```python
from build123d import *

# Parameters (mm, degrees)
F1_DEPTH = 9.525
F2_R     = 3.90906
F3_DEPTH = 25.4
F4_DEPTH = 25.4
F5_R     = 3.90525
F6_DEPTH = 25.4


# Not quite as in the source:
# - a fillet or chamfer that OpenCascade refuses, or shapes differently, is made with other operations: its cross-section is extruded or revolved along the edge and cut away or added


with BuildPart() as f1:
    # F0 (on Top) → F1 (new body, symmetric)
    with BuildSketch(Plane.XY):
        with BuildLine():
            Line((0, 20.6466445854), (-11.58875, 20.6466445854))
            ThreePointArc((-11.58875, 20.6466445854), (-17.1096965819, 19.861848606), (-22.19325, 17.5696355848))
            Line((-22.19325, 17.5696355848), (-22.19325, -17.5696355848))
            ThreePointArc((-22.19325, -17.5696355848), (-17.1096965819, -19.861848606), (-11.58875, -20.6466445854))
            Line((-11.58875, -20.6466445854), (0, -20.6466445854))
            Line((0, -20.6466445854), (11.58875, -20.6466445854))
            ThreePointArc((11.58875, -20.6466445854), (17.1096965819, -19.861848606), (22.19325, -17.5696355848))
            Line((22.19325, -17.5696355848), (22.19325, 17.5696355848))
            ThreePointArc((22.19325, 17.5696355848), (17.1096965819, 19.861848606), (11.58875, 20.6466445854))
            Line((11.58875, 20.6466445854), (0, 20.6466445854))
        make_face()
        with BuildLine():
            ThreePointArc((11.58875, 19.8846445854), (16.6970877606, 19.1869573913), (21.43125, 17.145))
            Line((21.43125, 17.145), (21.43125, -17.145))
            ThreePointArc((21.43125, -17.145), (16.6970877606, -19.1869573913), (11.58875, -19.8846445854))
            Line((11.58875, -19.8846445854), (0, -19.8846445854))
            Line((0, -19.8846445854), (-11.58875, -19.8846445854))
            ThreePointArc((-11.58875, -19.8846445854), (-16.6970877606, -19.1869573913), (-21.43125, -17.145))
            Line((-21.43125, -17.145), (-21.43125, 17.145))
            ThreePointArc((-21.43125, 17.145), (-16.6970877606, 19.1869573913), (-11.58875, 19.8846445854))
            Line((-11.58875, 19.8846445854), (0, 19.8846445854))
            Line((0, 19.8846445854), (11.58875, 19.8846445854))
        make_face(mode=Mode.SUBTRACT)
    extrude(amount=F1_DEPTH, both=True)

    # F2 (on face) → F3 (cut)
    with BuildSketch(Plane.YZ.offset(22.19325)):
        with BuildLine():
            ThreePointArc((0.396875, -6.3375855209), (4.6283180665, -4.3475478002), (6.35, 0))
            ThreePointArc((6.35, 0), (4.6283180665, 4.3475478002), (0.396875, 6.3375855209))
            Line((0.396875, 6.3375855209), (0.396875, -6.3375855209))
        make_face()
        with BuildLine():
            Line((0.396875, -6.3375855209), (0.396875, 6.3375855209))
            ThreePointArc((0.396875, 6.3375855209), (0, 6.35), (-0.396875, 6.3375855209))
            Line((-0.396875, 6.3375855209), (-0.396875, -6.3375855209))
            ThreePointArc((-0.396875, -6.3375855209), (0, -6.35), (0.396875, -6.3375855209))
        make_face()
        with BuildLine():
            ThreePointArc((-0.396875, 6.3375855209), (0, 6.35), (0.396875, 6.3375855209))
            Line((0.396875, 6.3375855209), (0.396875, 16.235569492))
            Line((0.396875, 16.235569492), (-0.396875, 16.235569492))
            Line((-0.396875, 16.235569492), (-0.396875, 6.3375855209))
        make_face()
        with BuildLine():
            Line((0.396875, -16.235569492), (0.396875, -6.3375855209))
            ThreePointArc((0.396875, -6.3375855209), (0, -6.35), (-0.396875, -6.3375855209))
            Line((-0.396875, -6.3375855209), (-0.396875, -16.235569492))
            Line((-0.396875, -16.235569492), (0.396875, -16.235569492))
        make_face()
        with BuildLine():
            Line((-0.396875, -6.3375855209), (-0.396875, 6.3375855209))
            ThreePointArc((-0.396875, 6.3375855209), (-6.35, 0), (-0.396875, -6.3375855209))
        make_face()
        with Locations((-11.9634, 0)):
            Circle(F2_R)
        with Locations((11.9634, 0)):
            Circle(F2_R)
    extrude(amount=-F3_DEPTH, mode=Mode.SUBTRACT)

    # F2 (on face) → F4 (cut)
    with BuildSketch(Plane.YZ.offset(22.19325)):
        with BuildLine():
            ThreePointArc((0.396875, -6.3375855209), (4.6283180665, -4.3475478002), (6.35, 0))
            ThreePointArc((6.35, 0), (4.6283180665, 4.3475478002), (0.396875, 6.3375855209))
            Line((0.396875, 6.3375855209), (0.396875, -6.3375855209))
        make_face()
        with BuildLine():
            Line((0.396875, -6.3375855209), (0.396875, 6.3375855209))
            ThreePointArc((0.396875, 6.3375855209), (0, 6.35), (-0.396875, 6.3375855209))
            Line((-0.396875, 6.3375855209), (-0.396875, -6.3375855209))
            ThreePointArc((-0.396875, -6.3375855209), (0, -6.35), (0.396875, -6.3375855209))
        make_face()
        with BuildLine():
            ThreePointArc((-0.396875, 6.3375855209), (0, 6.35), (0.396875, 6.3375855209))
            Line((0.396875, 6.3375855209), (0.396875, 16.235569492))
            Line((0.396875, 16.235569492), (-0.396875, 16.235569492))
            Line((-0.396875, 16.235569492), (-0.396875, 6.3375855209))
        make_face()
        with BuildLine():
            Line((0.396875, -16.235569492), (0.396875, -6.3375855209))
            ThreePointArc((0.396875, -6.3375855209), (0, -6.35), (-0.396875, -6.3375855209))
            Line((-0.396875, -6.3375855209), (-0.396875, -16.235569492))
            Line((-0.396875, -16.235569492), (0.396875, -16.235569492))
        make_face()
        with BuildLine():
            Line((-0.396875, -6.3375855209), (-0.396875, 6.3375855209))
            ThreePointArc((-0.396875, 6.3375855209), (-6.35, 0), (-0.396875, -6.3375855209))
        make_face()
        with Locations((-11.9634, 0)):
            Circle(F2_R)
        with Locations((11.9634, 0)):
            Circle(F2_R)
    extrude(amount=-F4_DEPTH, mode=Mode.SUBTRACT)

    # F5 (on face) → F6 (cut)
    with BuildSketch(Plane(origin=(-22.19325, 0, 0), x_dir=(0, -1, 0), z_dir=(-1, 0, 0))):
        Circle(F5_R)
    extrude(amount=-F6_DEPTH, mode=Mode.SUBTRACT)

    # F7: chamfer of 0.762 x 0.8765807263 on 3 edges, made by hand

    # F7_s1 → F7_t2 (revolve, cut)
    with BuildSketch(Plane.XY):
        Polygon((22.19325, -7.1777592737), (21.43125, -8.05434), (22.19325, -8.05434), align=None)
    revolve(axis=Axis((22.19325, -11.9634, 0), (1, 0, 0)), mode=Mode.SUBTRACT)

    # F7_s3 → F7_t4 (revolve, cut)
    with BuildSketch(Plane.XY):
        Polygon((22.19325, 16.63446), (21.3166692737, 15.87246), (22.19325, 15.87246), align=None)
    revolve(axis=Axis((22.19325, 11.9634, 0), (1, 0, 0)), mode=Mode.SUBTRACT)

    # F7_s5 → F7_t6 (revolve, cut)
    with BuildSketch(Plane.XY):
        Polygon((-22.19325, -4.7818307263), (-21.43125, -3.90525), (-22.19325, -3.90525), align=None)
    revolve(axis=Axis((-22.19325, 0, 0), (-1, 0, 0)), mode=Mode.SUBTRACT)


solid = f1.part
```
Work out the finished part from the listing and answer in its coordinate system (mm). A direction names the side the tool comes from. Give positions to 0.01 mm unless a question says otherwise; leave off trailing zeros. Loops run counter-clockwise (first coordinate to the right, second up) from the corner with the lowest first, then second, coordinate; pieces in that order, holes last. Notation, with made-up numbers: (48.5, 80.25) -> (57.5, 80.25) arc R24 ccw to (57.5, 109.25) -> close; hole circle Ø8 at (-35, -18). An arc over 180 degrees is marked (long way). Put each result on its own line as item: value. Start each with the question number.
Item 1: Find the intervals of material crossed by L1, parallel to X at y = 12, z = 7.5; L2, parallel to Y at x = 8.5, z = -5.5; L3, parallel to Y at x = -14, z = 2.25, in increasing order. Write a range as [from, to].
Item 2: The mould has two halves that part along X. Classify faces 4 (the face through (17.034, -19.884, 0.133)), 5 (the face through (21.431, 7, 0)), 6 (the face through (0, 20.647, 0)): released by +X, released by -X, zero draft, split by the parting line, or undercut.
Item 3: The part is cut by section A-A (x = 8). Give the vertices of the cut face in (y, z) (3 decimals).
Item 4: Which of the six approach directions +Z, -Z, +X, -X, +Y, -Y give full straight-line access (tool end or side, diameter ignored) to faces 1 (the face through (21.82, -6.35, 0.13)), 2 (the face through (-22.193, 4, 4)), 3 (the face through (-16.627, -19.206, 0.133))?
Item 5: Each of these flat-tipped pins is pushed along its axis until it touches: P1, Ø0.6, axis at x = 22, z = -8, coming from the +Y side; P2, Ø1, axis at x = -16.5, z = 3.5, coming from the +Y side. Where does it stop, or does it pass through?
Item 6: The part is cut by section B-B (y = 1). State how many separate pieces and enclosed holes the cut face has, then the cut area to 3 significant figures.
Answers below:
1. L1: [-22.19, -21.43], [21.43, 22.19]
1. L2: [-20.65, -19.88], [19.88, 20.65]
1. L3: [-20.5, -19.73], [19.73, 20.5]
2. face 4: released by +X
2. face 5: undercut
2. face 6: zero draft
3. outline: (-20.647, -9.525) -> (-19.885, -9.525) -> (-19.885, 9.525) -> (-20.647, 9.525) -> close; (19.885, -9.525) -> (20.647, -9.525) -> (20.647, 9.525) -> (19.885, 9.525) -> close
4. face 1: +X
4. face 2: +Z, -Z, -X, +Y, -Y
4. face 3: +Z, -Z
5. P1: y = 17.87
5. P2: y = 20.15
6. separate pieces: 4
6. enclosed holes: 0
6. area: 13.0 mm2
